Check sheet for the modelled part. Datum: model origin and axes. Units: mm. A direction names the side the tool comes from. Coordinates: 2 decimals unless noted, no trailing zeros. Write each loop counter-clockwise with the first axis right and the second up, starting at its lowest first coordinate (ties: lowest second). Pieces come first, ordered by that corner, then holes. Notation, with made-up numbers: (50, -26) - (76, -26) arc R15 ccw to (76, -18) - close; hole circle Ø6 at (87, 55). An arc over 180 degrees is marked (long way). Write each question's results on one line, items separated by ' | '.
from build123d import *

# Parameters (mm, degrees)
SKETCH_1_R               = 2
SKETCH_1_R_2             = 1.5
EXTRUDE_1_DEPTH          = 8
CUT_EXTRUDE_1_DEPTH      = 9
SKETCH_3_R               = 2.5
CUT_EXTRUDE_2_DEPTH      = 1
CUT_EXTRUDE_2_DEPTH_BACK = 9


with BuildPart() as part:
    # 草图1 → 凸台-拉伸1 (new body)
    with BuildSketch(Plane(origin=(0, 0, 0), x_dir=(1, 0, 0), z_dir=(0, 1, 0))):
        with BuildLine():
            Line((0, 19.5), (127.428932188, 19.5))
            ThreePointArc((127.428932188, 19.5), (132.048329851, 16.413417162), (130.964466094, 10.964466094))
            Line((130.964466094, 10.964466094), (103.428932188, -16.571067812))
            ThreePointArc((103.428932188, -16.571067812), (100.1846987, -18.738795325), (96.357864376, -19.5))
            Line((96.357864376, -19.5), (0, -19.5))
            ThreePointArc((0, -19.5), (-19.5, 0), (0, 19.5))
        make_face()
        with Locations((0, 12.15)):
            Circle(SKETCH_1_R, mode=Mode.SUBTRACT)
        with Locations((-10.522208656, -6.075)):
            Circle(SKETCH_1_R, mode=Mode.SUBTRACT)
        with Locations((10.522208656, -6.075)):
            Circle(SKETCH_1_R, mode=Mode.SUBTRACT)
        with Locations((-11.691342951, 6.75)):
            Circle(SKETCH_1_R_2, mode=Mode.SUBTRACT)
        with Locations((11.691342951, 6.75)):
            Circle(SKETCH_1_R_2, mode=Mode.SUBTRACT)
        with Locations((0, -13.5)):
            Circle(SKETCH_1_R_2, mode=Mode.SUBTRACT)
    extrude(amount=EXTRUDE_1_DEPTH)

    # 草图2 → 切除-拉伸1 (cut, through all)
    with BuildSketch(Plane.XZ):
        with BuildLine():
            Line((93.872583002, 7.5), (74.902020254, 7.5))
            ThreePointArc((74.902020254, 7.5), (73.054261189, 6.265366865), (73.487806691, 4.085786438))
            Line((73.487806691, 4.085786438), (83.902020254, -6.328427125))
            ThreePointArc((83.902020254, -6.328427125), (85.199713649, -7.19551813), (86.730447378, -7.5))
            Line((86.730447378, -7.5), (105.701010127, -7.5))
            ThreePointArc((105.701010127, -7.5), (107.548769192, -6.265366865), (107.115223689, -4.085786438))
            Line((107.115223689, -4.085786438), (96.701010127, 6.328427125))
            ThreePointArc((96.701010127, 6.328427125), (95.403316731, 7.19551813), (93.872583002, 7.5))
        make_face()
    extrude(amount=-CUT_EXTRUDE_1_DEPTH, mode=Mode.SUBTRACT)

    # 草图3 → 切除-拉伸2 (cut, two sides)
    with BuildSketch(Plane.XZ) as cut_extrude_2_sk:
        with Locations((97.600505063, 12.5)):
            Circle(SKETCH_3_R)
        with Locations((122.600505063, -12.5)):
            Circle(SKETCH_3_R)
        with Locations((83.002525317, -12.5)):
            Circle(SKETCH_3_R)
        with Locations((58.002525317, 12.5)):
            Circle(SKETCH_3_R)
    extrude(amount=CUT_EXTRUDE_2_DEPTH, mode=Mode.SUBTRACT)
    extrude(cut_extrude_2_sk.sketch, amount=-CUT_EXTRUDE_2_DEPTH_BACK, mode=Mode.SUBTRACT)


solid = part.part
1. Sectioned sample at D-D (x = -3.5). Record the cut outline in (y, z).
Values follow:
outline: (0, -19.18) - (8, -19.18) - (8, 19.18) - (0, 19.18) - close
2. Access from +Z, -Z, +X, -X, +Y, -Y to the whole of each face (thin tool, end or side, straight path). Record for faces 1 (the cylindrical face through (107.536, 3.944, -6.296)), 2 (the flat face through (117, 4, 3)).
Values follow:
face 1: +Y, -Y | face 2: +Z, +X, +Y, -Y
3. Material ranges on L1, parallel to Z at x = 93.5, y = 6.75; L2, parallel to X at y = 1.75, z = 11.5; L3, parallel to X at y = 4, z = -7, recorded low to high. Write a range as [from, to].
Values follow:
L1: z = [-19.5, -7.5], [7.5, 19.5] | L2: x = [-15.75, 55.71], [60.29, 95.31], [99.89, 108.5] | L3: x = [-18.2, -13.17], [-10.21, 10.21], [13.17, 84.79], [107.02, 127]
4. Sectioned sample at C-C (y = 5.75). Give the number of separate pieces and of enclosed holes in the cut face, then the cut area to 3 significant figures.
Values follow:
separate pieces: 1 | enclosed holes: 11 | area: 4,740 mm^2
5. Draft check along Z on faces 3 (the flat face through (58, 8, 0)), 4 (the flat face through (78.622, 3.944, -1.048)), 5 (the flat face through (63, 4, -19.5)). Enter one of: pulls with the +Z half, pulls with the -Z half, needs draft (parallel to the pull), parting line crosses it, or undercut.
Values follow:
face 3: needs draft | face 4: undercut | face 5: pulls with the -Z half
6. Sectioned sample at A-A (x = 90). Record the cut outline in (y, z).
Values follow:
outline: (0, -19.5) - (8, -19.5) - (8, -7.5) - (0, -7.5) - close; (0, 7.5) - (8, 7.5) - (8, 19.5) - (0, 19.5) - close
7. Go/stop test with a flat-tipped pin: pin 1 (1 mm diameter, centred on y = 7, z = 10.5, fed in from +X). Record where the tip stops, or that it passes through.
Values follow:
pin 1: stops at x = 110
8. Sectioned sample at B-B (z = 1). Record the cut outline in (x, y), then the cut area to 3 significant figures.
Values follow:
outline: (-19.47, 0) - (76.57, 0) - (76.57, 8) - (-19.47, 8) - close; (102.03, 0) - (119, 0) - (119, 8) - (102.03, 8) - close | area: 904 mm^2
